from build123d import *

# Parameters (mm, degrees)
SKETCH1_W           = 4
SKETCH1_H           = 8
BOSS_EXTRUDE1_DEPTH = 10
CHAMFER1_SIZE       = 0.5


with BuildPart() as part:
    # Sketch1 → Boss-Extrude1 (new body)
    with BuildSketch(Plane.XY):
        Rectangle(SKETCH1_W, SKETCH1_H)
    extrude(amount=BOSS_EXTRUDE1_DEPTH)

    # Chamfer1
    chamfer1_edges = [part.edges().sort_by_distance(p)[0] for p in [
        (2, -4, 5),
        (-2, -4, 5),
        (-2, 4, 5),
        (2, 4, 5),
    ]]
    chamfer(chamfer1_edges, length=CHAMFER1_SIZE)


solid = part.part
Work out the finished part from the listing and answer in its coordinate system (mm). Give positions to 0.01 mm unless a question says otherwise; leave off trailing zeros. Order: outer loops, then holes, each group sorted by start corner. A loop starts at its lowest first (then second) coordinate and runs counter-clockwise, first axis right, second up. Notation, with made-up numbers: (28, 53.5) -> (41, 53.5) arc R26 ccw to (41, 84.5) -> close; hole circle Ø6 at (-1, 32.5). An arc over 180 degrees is marked (long way). Answer as a JSON object with one key per item and string values. Group by question number.
1. Section A-A on z = 2.5 is taken. Determine the outline of the cut face in (x, y), plus the area to 3 significant figures.
2. Consider line 1 along Y through (x, z) = (1.65, 5.25). Determine where the line is inside the solid, lowest interval first. Write a range as [from, to].
3. Section B-B on x = 1.75 is taken. Determine the outline of the cut face in (y, z), plus the area to 3 significant figures.
Result sheet:
{
 "1": {"outline": "(-2, -3.5) -> (-1.5, -4) -> (1.5, -4) -> (2, -3.5) -> (2, 3.5) -> (1.5, 4) -> (-1.5, 4) -> (-2, 3.5) -> close", "area": "31.5 mm^2"},
 "2": {"line 1": "y = [-3.85, 3.85]"},
 "3": {"outline": "(-3.75, 0) -> (3.75, 0) -> (3.75, 10) -> (-3.75, 10) -> close", "area": "75.0 mm^2"}
}
